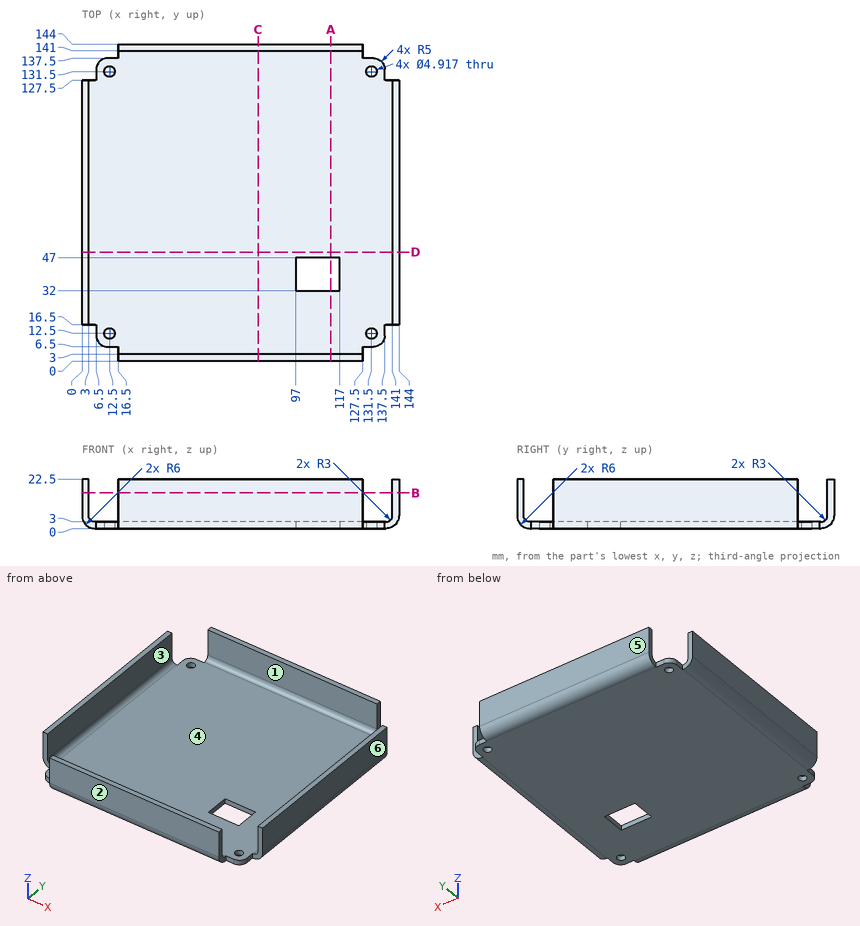
Geometry check sheet. Reference: drawing and pictorial views, mm from the part's lowest x, y, z. A direction names the side the tool comes from. Round coordinates to 2 decimals unless told otherwise and drop trailing zeros. Write each loop counter-clockwise with the first axis right and the second up, starting at its lowest first coordinate (ties: lowest second). Pieces come first, ordered by that corner, then holes.
Item 1: Material ranges on line 1 along Y through (x, z) = (131.5, 1.95); line 2 along X through (y, z) = (52.5, 17.5), recorded low to high.
Determined:
line 1: y = 6.5 to 10.04, 14.96 to 129.04, 133.96 to 137.5
line 2: x = 0 to 3, 141 to 144
Item 2: Section check B-B (z = 16.25). Record the boundary of the cut face in (x, y).
Determined:
outline: (0, 16.5) - (3, 16.5) - (3, 127.5) - (0, 127.5) - close; (16.5, 0) - (127.5, 0) - (127.5, 3) - (16.5, 3) - close; (16.5, 141) - (127.5, 141) - (127.5, 144) - (16.5, 144) - close; (141, 16.5) - (144, 16.5) - (144, 127.5) - (141, 127.5) - close
Item 3: Mould release check, pull along Y, two halves, no side actions. Record for the marked faces 4, 5 and 6: +Y half, -Y half, draft (parallel to the pull), parting line (faces both ways), or undercut.
Determined:
face 4: undercut
face 5: +Y half
face 6: draft
Item 4: Section check C-C (x = 80). Record the boundary of the cut face in (y, z).
Determined:
outline: (0, 6) arc R6 ccw to (6, 0) - (138, 0) arc R6 ccw to (144, 6) - (144, 22.5) - (141, 22.5) - (141, 6) arc R3 cw to (138, 3) - (6, 3) arc R3 cw to (3, 6) - (3, 22.5) - (0, 22.5) - close
Item 5: Section check A-A (x = 113). Record the boundary of the cut face in (y, z).
Determined:
outline: (0, 6) arc R6 ccw to (6, 0) - (32, 0) - (32, 3) - (6, 3) arc R3 cw to (3, 6) - (3, 22.5) - (0, 22.5) - close; (47, 0) - (138, 0) arc R6 ccw to (144, 6) - (144, 22.5) - (141, 22.5) - (141, 6) arc R3 cw to (138, 3) - (47, 3) - close
Item 6: Go/stop test with flat-tipped pins: pin 1 Ø2.5 at (x, z) = (14, 2) entering from -Y; pin 2 Ø3.5 at (x, z) = (108.5, 1.5) entering from -Y; pin 3 Ø12 at (x, y) = (114.5, 14.5) entering from +Z; pin 4 Ø3 at (x, z) = (5, 12.5) entering from -Y. Record where each tip stops, or that it passes through.
Determined:
pin 1: stops at y = 6.5
pin 2: stops at y = 0.67
pin 3: stops at z = 3
pin 4: passes through
Item 7: Access from +Z, -Z, +X, -X, +Y, -Y to the whole of each face (thin tool, end or side, straight path). Record for the marked faces 1, 2 and 3.
Determined:
face 1: +Z, +X, -X
face 2: +Z, -Z, +X, -X, -Y
face 3: +Z, +Y, -Y
